Autodesk Inventor part; units mm, degrees
ref_plane "Work Plane1" through (6.35, 0, 0) normal (1, 0, 0) x (0, 1, 0)
ref_plane "Work Plane2" through (0, 0, -6.35) normal (0, 0, 1) x (1, 0, 0)
ref_plane "XZ Plane" through (0, 0, 0) normal (0, 1, 0) x (-1, 0, 0)
sketch "Sketch1" plane through (0, 0, 0) normal (0, 1, 0) x (-1, 0, 0)
  line L0 (0, 0) -> (41.275, 0)
  line L1 (41.275, -2.54) -> (0, -2.54)
  line L2 (41.275, -2.54) -> (41.275, 0)
  dimension "d69" = 41.275
  dimension "d70" = 41.275
  dimension "d89" = 2.54
  dimension "d90" = 0
  dimension "d91" = 0
  dimension "d92" = 0
sketch "Sketch2" plane through (0, 0, 0) normal (1, 0, 0) x (0, 1, 0)
  line L0 (0, 0) -> (0.254, 0)
  line L1 (0.254, 0) -> (0.254, -0.254)
  line L2 (0.254, -0.254) -> (0, -0.254)
  line L3 (0, -0.254) -> (0, 0)
  dimension "d98" = 0.254
  dimension "d99" = 0.254
sweep "Sweep1" add profiles "Sketch2" path "Sketch1"
ref_plane "Work Plane1" through (6.35, 0, 0) normal (1, 0, 0) x (0, 1, 0)
ref_plane "Work Plane2" through (0, 0, -6.35) normal (0, 0, 1) x (1, 0, 0)
ref_plane "Work Plane4" through (0, 0, -2.9845) normal (0, 0, 1) x (1, 0, 0)
properties part number "abs_1_loop" material "Silver"
Geometry: final body of the model. Coordinates: model frame, mm. Round coordinates to 2 decimals unless told otherwise and drop trailing zeros. Loops run counter-clockwise (first coordinate to the right, second up) from the corner with the lowest first, then second, coordinate; pieces in that order, holes last. Notation, with made-up numbers: (11.5, 66) - (39.5, 66) arc R20 ccw to (39.5, 95) - close; hole circle Ø3 at (-33, 88). An arc over 180 degrees is marked (long way). Write each question's results on one line, items separated by ' | '. Start each with the question number.
1) Cut plane A-A on x = -12. Return loops of the section in (y, z), then the cut area to 3 significant figures.
2) Cut plane C-C on z = -0.8. Return loops of the section in (x, y) (3 decimals), then the cut area to 3 significant figures.
3) Line query: probe 1 along Z at (x, y) = (-8.5, 0.15); probe 2 along X at (y, z) = (0.15, -1.8) (3 decimals). Output: solid intervals per line, ascending. Write a range as [from, to].
4) Cut plane B-B on y = 0.1. Return loops of the section in (x, z) (3 decimals), then the cut area to 3 significant figures.
Verdict:
1) outline: (0, -2.54) - (0.25, -2.54) - (0.25, -2.29) - (0, -2.29) - close; (0, -0.25) - (0.25, -0.25) - (0.25, 0) - (0, 0) - close | area: 0.129 mm2
2) outline: (-41.275, 0) - (-41.021, 0) - (-41.021, 0.254) - (-41.275, 0.254) - close | area: 0.0645 mm2
3) probe 1: z = [-2.54, -2.29], [-0.25, 0] | probe 2: x = [-41.275, -41.021]
4) outline: (-41.275, -2.54) - (0, -2.54) - (0, -2.286) - (-41.021, -2.286) - (-41.021, -0.254) - (0, -0.254) - (0, 0) - (-41.275, 0) - close | area: 21.5 mm2
